from build123d import *

# Parameters (mm, degrees)
F1_DEPTH = 48.26
F3_DEPTH = 25.4
F4_R     = 2.54


with BuildPart() as f1:
    # F0 (on Top) → F1 (new body)
    with BuildSketch(Plane.XY):
        with BuildLine():
            Line((0, -50.8), (63.5, -50.8))
            Line((63.5, -50.8), (63.5, -18.4782915836))
            ThreePointArc((63.5, -18.4782915836), (110.0348201001, 70.4604594113), (38.5441593826, 0))
            Line((38.5441593826, 0), (0, 0))
            Line((0, 0), (0, -50.8))
        make_face()
    extrude(amount=F1_DEPTH)

    # F2 (on face) → F3 (intersect)
    with BuildSketch(Plane.XY.offset(48.26)):
        with BuildLine():
            ThreePointArc((63.5, -18.4782915836), (110.0348201001, 70.4604594113), (38.5441593826, 0))
            Line((38.5441593826, 0), (0, 0))
            Line((0, 0), (0, -50.8))
            Line((0, -50.8), (63.5, -50.8))
            Line((63.5, -50.8), (63.5, -18.4782915836))
        make_face()
        Polygon((81.7504222175, 3.7261128257), (55.766562748, 19.7779196896), (63.0032841086, 49.4503196679), (93.4596833462, 51.7370645185), (105.0460518893, 23.4779505813), align=None, mode=Mode.SUBTRACT)
    extrude(amount=-F3_DEPTH, mode=Mode.INTERSECT)

    # F4
    f4_edges = [f1.edges().sort_by_distance(p)[0] for p in [
        (110.03482, 70.460459, 48.26),
        (19.27208, 0, 48.26),
        (0, -25.4, 48.26),
        (63.5, -34.639146, 48.26),
        (31.75, -50.8, 48.26),
        (99.252868, 37.607508, 48.26),
        (78.231484, 50.593692, 48.26),
        (59.384923, 34.61412, 48.26),
        (68.758492, 11.752016, 48.26),
        (93.398237, 13.602032, 48.26),
    ]]
    fillet(f4_edges, radius=F4_R)


solid = f1.part
Could you check a few things on this model? Use its own coordinates, in mm. A direction names the side the tool comes from. Give positions to 0.01 mm unless a question says otherwise; leave off trailing zeros. Order: outer loops, then holes, each group sorted by start corner. A loop starts at its lowest first (then second) coordinate and runs counter-clockwise, first axis right, second up.
1. Suppose I cut it at B-B (y = -39). Write out the boundary of the cut face in (x, z).
Answers below:
outline: (0, 22.86) - (63.5, 22.86) - (63.5, 45.72) arc R2.54 ccw to (60.96, 48.26) - (2.54, 48.26) arc R2.54 ccw to (0, 45.72) - close
2. Which directions (+Z, -Z, +X, -X, +Y, -Y) give clear straight access to the entire face, cutting with the end or side of a thin tool? Please do faces 5 (the flat face through (99.17, 37.81, 34.45)), 6 (the flat face through (20, 0, 34)), 7 (the cylindrical face through (100, 37.7, 47.5)).
Answers below:
face 5: +Z, -Z
face 6: +Z, -Z, -X
face 7: +Z
3. Suppose I cut it at C-C (x = 21). Write out the boundary of the cut face in (y, z), plus the area to 3 significant figures.
Answers below:
outline: (-50.8, 22.86) - (0, 22.86) - (0, 45.72) arc R2.54 ccw to (-2.54, 48.26) - (-48.26, 48.26) arc R2.54 ccw to (-50.8, 45.72) - close
area: 1,290 mm2
4. For pin 1 (6 mm diameter, centred on x = 85, z = 31, fed in from +Y); pin 2 (4 mm diameter, centred on x = 14.5, z = 29.5, fed in from +Y); pin 3 (1 mm diameter, centred on x = 71, y = -21.5, fed in from -Z); pin 4 (1 mm diameter, centred on y = 21, z = 42.5, fed in from +X), each with a flat end and sliding along its axis, tell me the tip position at first contact or that it passes through.
Answers below:
pin 1: stops at y = 80.39
pin 2: stops at y = 0
pin 3: passes through
pin 4: stops at x = 129.95
5. I need wall thicknesses on L1, parallel to Y at x = 8, z = 24; L2, parallel to X at y = 44, z = 29; L3, parallel to X at y = -34, z = 34.5. Which ranges of each line are inside material? Lowest first, please.
Answers below:
L1: y = -50.8 to 0
L2: x = 31.08 to 61.67, 96.63 to 128.53
L3: x = 0 to 63.5
6. Thinking about a two-plate mould opening in X: for faces 1 (the flat face through (0, -25, 34)), 2 (the flat face through (59.334, 34.406, 34.45)), 3 (the flat face through (64, 1, 22.86)), 4 (the cylindrical face through (93.7, 12.9, 47.5)), which applies, +X half, -X half, draft (parallel to the pull), parting line (faces both ways), or undercut?
Answers below:
face 1: -X half
face 2: undercut
face 3: draft
face 4: undercut
7. Suppose I cut it at A-A (z = 31.5). Write out the boundary of the cut face in (x, y).
Answers below:
outline: (0, -50.8) - (63.5, -50.8) - (63.5, -18.48) arc R50.8 ccw (long way) to (38.54, 0) - (0, 0) - close; hole (55.77, 19.78) - (81.75, 3.73) - (105.05, 23.48) - (93.46, 51.74) - (63, 49.45) - close
